Here's the drawing with two shaded views (mm, measured from the low corner). I have some questions. Round coordinates to 2 decimals unless told otherwise and drop trailing zeros. Order: outer loops, then holes, each group sorted by start corner. A loop starts at its lowest first (then second) coordinate and runs counter-clockwise, first axis right, second up.
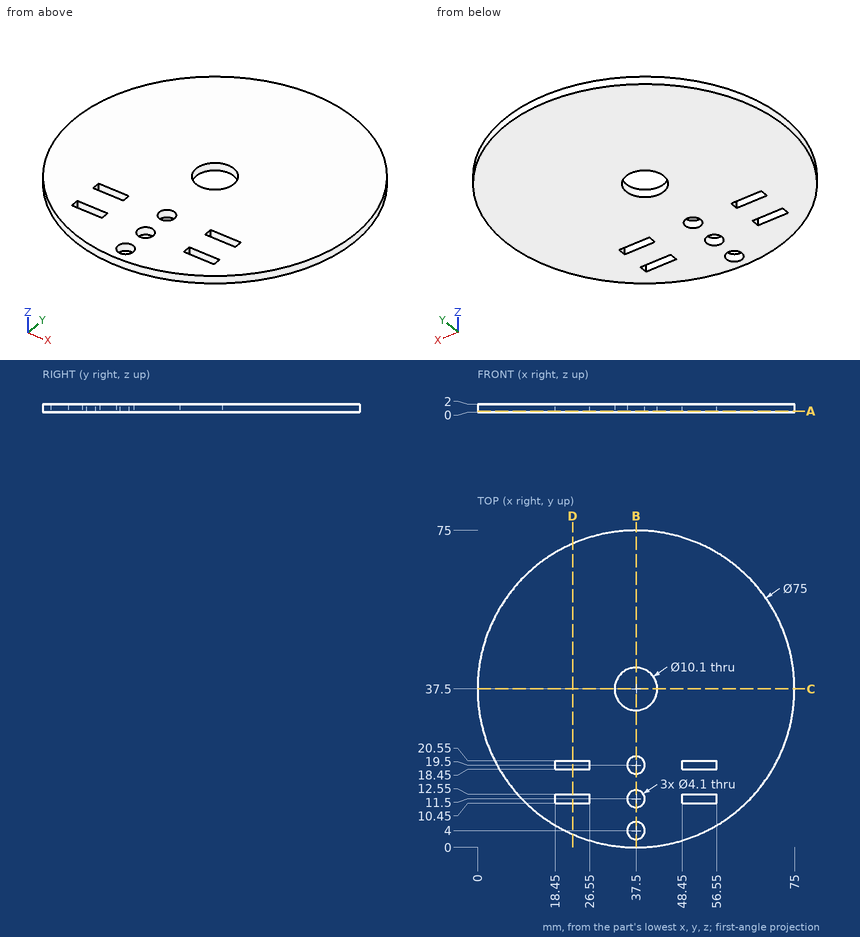
1. If we section it at D-D, the plane x = 22.5: Write out the boundary of the cut face in (y, z).
Evaluation:
outline: (3.13, 0) - (10.45, 0) - (10.45, 2) - (3.13, 2) - close; (12.55, 0) - (18.45, 0) - (18.45, 2) - (12.55, 2) - close; (20.55, 0) - (71.87, 0) - (71.87, 2) - (20.55, 2) - close
2. I need wall thicknesses on probe 1 along Y at (x, z) = (37.5, 1.4); probe 2 along X at (y, z) = (56.5, 0.6); probe 3 along Y at (x, z) = (48, 0.75). Which ranges of each line are inside material? Lowest first, please.
Evaluation:
probe 1: y = 0 to 1.95, 6.05 to 9.45, 13.55 to 17.45, 21.55 to 32.45, 42.55 to 75
probe 2: x = 5.17 to 69.83
probe 3: y = 1.5 to 73.5
3. If we section it at B-B, the plane x = 37.5: Write out the boundary of the cut face in (y, z).
Evaluation:
outline: (0, 0) - (1.95, 0) - (1.95, 2) - (0, 2) - close; (6.05, 0) - (9.45, 0) - (9.45, 2) - (6.05, 2) - close; (13.55, 0) - (17.45, 0) - (17.45, 2) - (13.55, 2) - close; (21.55, 0) - (32.45, 0) - (32.45, 2) - (21.55, 2) - close; (42.55, 0) - (75, 0) - (75, 2) - (42.55, 2) - close
4. If we section it at A-A, the plane z = 0.3: State how many separate pieces and enclosed holes the cut face has, and give its area (3 significant figures).
Evaluation:
separate pieces: 1
enclosed holes: 8
area: 4,230 mm2
5. I'm going to push flat-ended pins straight in: P1, Ø0.6, axis at y = 11, z = 0.5, coming from the +X side; P2, Ø1, axis at y = 19.5, z = 0.5, coming from the +X side; P3, Ø1, axis at x = 53, z = 1.5, coming from the -Y side. Where does each tip first touch, or does it pass through?
Evaluation:
P1: stops at x = 64.33
P2: stops at x = 70.67
P3: stops at y = 3.13
6. If we section it at C-C, the plane y = 37.5: Write out the boundary of the cut face in (x, z), and give its area (3 significant figures).
Evaluation:
outline: (0, 0) - (32.45, 0) - (32.45, 2) - (0, 2) - close; (42.55, 0) - (75, 0) - (75, 2) - (42.55, 2) - close
area: 130 mm2
